from build123d import *

# Parameters (mm, degrees)
F1_DEPTH    = 25.4
F2_DEPTH    = 22.098
F3_T1_DEPTH = 495.3


# Not quite as in the source:
# - a fillet or chamfer that OpenCascade refuses, or shapes differently, is made with other operations: its cross-section is extruded or revolved along the edge and cut away or added


with BuildPart() as f1:
    # F0 (on Top) → F1 (new body)
    with BuildSketch(Plane.XY):
        with BuildLine():
            ThreePointArc((215.9, -82.55), (220.7013488144, -81.6074252948), (224.79, -78.9196141042))
            Line((224.79, -78.9196141042), (224.79, -69.85))
            Line((224.79, -69.85), (224.79, 69.85))
            ThreePointArc((224.79, 69.85), (222.1861792847, 76.1361792847), (215.9, 78.74))
            Line((215.9, 78.74), (-215.9, 78.74))
            ThreePointArc((-215.9, 78.74), (-222.1861792847, 76.1361792847), (-224.79, 69.85))
            Line((-224.79, 69.85), (-224.79, -69.85))
            Line((-224.79, -69.85), (-224.79, -78.9196141042))
            ThreePointArc((-224.79, -78.9196141042), (-220.7013488144, -81.6074252948), (-215.9, -82.55))
            Line((-215.9, -82.55), (215.9, -82.55))
        make_face()
    extrude(amount=F1_DEPTH)

    # F0 (on Top) → F2 (join)
    with BuildSketch(Plane.XY):
        with BuildLine():
            ThreePointArc((228.6, 69.85), (224.8802561211, 78.8302561211), (215.9, 82.55))
            Line((215.9, 82.55), (-215.9, 82.55))
            ThreePointArc((-215.9, 82.55), (-224.8802561211, 78.8302561211), (-228.6, 69.85))
            ThreePointArc((-228.6, 69.85), (-230.7318859092, 0), (-228.6, -69.85))
            ThreePointArc((-228.6, -69.85), (-227.6088214608, -74.7686888497), (-224.79, -78.9196141042))
            Line((-224.79, -78.9196141042), (-224.79, -69.85))
            Line((-224.79, -69.85), (-224.79, 69.85))
            ThreePointArc((-224.79, 69.85), (-222.1861792847, 76.1361792847), (-215.9, 78.74))
            Line((-215.9, 78.74), (215.9, 78.74))
            ThreePointArc((215.9, 78.74), (222.1861792847, 76.1361792847), (224.79, 69.85))
            Line((224.79, 69.85), (224.79, -69.85))
            Line((224.79, -69.85), (224.79, -78.9196141042))
            ThreePointArc((224.79, -78.9196141042), (227.6088214608, -74.7686888497), (228.6, -69.85))
            ThreePointArc((228.6, -69.85), (230.9555402084, 0), (228.6, 69.85))
        make_face()
    extrude(amount=F2_DEPTH)

    # F3: fillet of radius 12.7 on 4 edges, made by hand

    # F3_s2 → F3_t1 (cut)
    with BuildSketch(Plane.YZ.offset(-247.65)):
        with BuildLine():
            add(Edge.make_bspline(
                [(-69.85, 0), (-82.55, 0), (-82.55, 12.7)],
                knots=[0, 0, 0, 1, 1, 1], degree=2, weights=[1, 1, 1]))
            Line((-82.55, 12.7), (-82.55, 0))
            Line((-82.55, 0), (-69.85, 0))
        make_face()
        with BuildLine():
            add(Edge.make_bspline(
                [(-69.85, 25.4), (-82.55, 25.4), (-82.55, 12.7)],
                knots=[0, 0, 0, 1, 1, 1], degree=2, weights=[1, 1, 1]))
            Line((-82.55, 12.7), (-82.55, 25.4))
            Line((-82.55, 25.4), (-69.85, 25.4))
        make_face()
    extrude(amount=F3_T1_DEPTH, mode=Mode.SUBTRACT)


solid = f1.part
Source: CAD feature listing. Evaluate the final solid. Frame: model axes, mm. A direction names the side the tool comes from. Coordinates: 2 decimals unless noted, no trailing zeros. Write each question's results on one line, items separated by ' | '. Start each with the question number.
1. Material intervals for L1, parallel to Y at x = -173, z = 14.5; L2, parallel to X at y = 9.5, z = 8.5; L3, parallel to Y at x = -127, z = 2.75, sorted ascending.
2. Reachability of faces 1 (the face through (-3, 7, 0)), 2 (the face through (-222.12, 76.2, 23.73)), 3 (the face through (222.25, 76.07, 23.73)) from +Z, -Z, +X, -X, +Y, -Y: full face, straight path, thin tool, end or side. Return the list, or none.
3. Pin query (flat end, axial travel): pin 1 (1.7 mm diameter, centred on y = -26.5, z = 23.5, fed in from +X); pin 2 (3.5 mm diameter, centred on y = -16, z = 23.5, fed in from -X); pin 3 (1 mm diameter, centred on x = 16.5, z = 23, fed in from +Y). Return the tip coordinate at first contact, or that it passes through.
Solution:
1) L1: -82.48 to 82.55 | L2: -230.69 to 230.91 | L3: -78.92 to 82.55
2) face 1: -Z, +X, -X, +Y, -Y | face 2: +Z, -X, +Y | face 3: +Z, +X, +Y
3) pin 1: x = 224.79 | pin 2: x = -230.63 | pin 3: y = 78.74
